Model file for the job. Use its own axes, mm. A direction names the side the tool comes from. Coordinates: 2 decimals unless noted, no trailing zeros. Order: outer loops, then holes, each group sorted by start corner. A loop starts at its lowest first (then second) coordinate and runs counter-clockwise, first axis right, second up. Notation, with made-up numbers: (70.25, -7) -> (78.25, -7) arc R21 ccw to (78.25, 28) -> close; hole circle Ø1 at (28.25, 56.25). An arc over 180 degrees is marked (long way). Return JSON: item names as keys, results as strings. Group by question number.
1) Cut at B-B (x = 26). Write the cut outline in (y, z), and give its area (3 significant figures).
2) Which spindle directions (+Z, -Z, +X, -X, +Y, -Y) get a long thin tool onto all of the face, cutting with end or side? Do faces 1 (the cylindrical face through (5.697, 48.008, 2.877)), 2 (the flat face through (1.016, 58, -11)), 3 (the flat face through (10, 11.43, -7)). Say none if no direction does.
3) Pull direction X, two halves, no side cores. Call faces 4 (the cylindrical face through (5.948, 49.785, -11.13)), 5 (the flat face through (-10, 61.976, 0)), 6 (the flat face through (37.846, 24, -2)): +X half, -X half, draft (parallel to the pull), parting line (faces both ways), or undercut.
4) Flat gauge pins, fed straight in: pin 1 (2 mm diameter, centred on x = 33.09, y = 58.03, fed in from -Z); pin 2 (3 mm diameter, centred on y = 7.5, z = -16, fed in from -X); pin 3 (2.5 mm diameter, centred on x = 13, z = 13, fed in from +Y); pin 4 (2.5 mm diameter, centred on x = -1.5, z = -7, fed in from +Y). Where does each tip first touch, or does it go through?
5) Cut at A-A (y = 26). Write the cut outline in (x, z).
6) Probe line 1 (Z direction, x = 24.5, y = 37); line 2 (X direction, y = 57, z = 4.5); line 3 (Y direction, x = -14.5, z = 12). List the from-to ranges inside material, lowest first.
from build123d import *

# Parameters (mm, degrees)
SKETCH1_W                       = 56.896
SKETCH1_H                       = 9.525
BOSS_EXTRUDE1_DEPTH             = 61.976
SKETCH2_R                       = 13.3985
CUT_EXTRUDE1_DEPTH              = 5.8801
CUT_EXTRUDE1_DRAFT              = -50
SKETCH5_W                       = 56.896
SKETCH5_H                       = 11.43
BOSS_EXTRUDE2_DEPTH             = 7.62
TAP_DRILL_FOR_M3X0_5_TAP3_D     = 2.5
TAP_DRILL_FOR_M3X0_5_TAP3_DEPTH = 25.4
TAP_DRILL_FOR_M3X0_5_TAP3_TIP   = 0.751075774
BOSS_EXTRUDE4_DEPTH             = 56.896
M3_CLEARANCE_HOLE3_D            = 3.7
M3_CLEARANCE_HOLE3_DEPTH        = 25.4
M3_CLEARANCE_HOLE3_TIP          = 1.111592145
SKETCH6_W                       = 56.896
SKETCH6_H                       = 2.54
BOSS_EXTRUDE5_DEPTH             = 50.546
SKETCH24_R                      = 4.826
CUT_EXTRUDE2_DEPTH              = 2.54
SKETCH25_R                      = 6.604
CUT_EXTRUDE3_DEPTH              = 7.366
M3_CLEARANCE_HOLE4_D            = 3.7
M3_CLEARANCE_HOLE4_DEPTH        = 17.272
M3_CLEARANCE_HOLE4_TIP          = 1.111592145


with BuildPart() as part:
    # Sketch1 → Boss-Extrude1 (new body)
    with BuildSketch(Plane(origin=(0, 0, 0), x_dir=(1, 0, 0), z_dir=(0, 1, 0))):
        with Locations((9.398, 0)):
            Rectangle(SKETCH1_W, SKETCH1_H)
    extrude(amount=BOSS_EXTRUDE1_DEPTH)


with BuildPart() as cut_extrude1_tool:
    # Sketch2 → Cut-Extrude1 (with draft: the straight prism first)
    with BuildSketch(Plane(origin=(0, 0, -4.7625), x_dir=(-1, 0, 0), z_dir=(0, 0, -1))):
        with Locations((-5.842, 54.552080914)):
            Circle(SKETCH2_R)
    extrude(amount=-CUT_EXTRUDE1_DEPTH)
    # Cut-Extrude1: the draft: its side faces are tilted about the plane it starts from
    cut_extrude1_sides = [cut_extrude1_tool.faces().sort_by_distance(p)[0] for p in [
        (19.2405, 54.552080914, -1.82245),
    ]]
    draft(cut_extrude1_sides, Plane(origin=(0, 0, -4.7625), x_dir=(-1, 0, 0), z_dir=(0, 0, -1)), CUT_EXTRUDE1_DRAFT)


with BuildPart() as part_1:
    add(part.part)

    # Cut-Extrude1: cut by cut_extrude1_tool
    add(cut_extrude1_tool.part, mode=Mode.SUBTRACT)

    # Sketch5 → Boss-Extrude2 (add)
    with BuildSketch(Plane(origin=(0, 0, -4.7625), x_dir=(-1, 0, 0), z_dir=(0, 0, -1))):
        with Locations((-9.398, 5.715)):
            Rectangle(SKETCH5_W, SKETCH5_H)
    extrude(amount=BOSS_EXTRUDE2_DEPTH)

    # Tap Drill for M3x0.5 Tap3
    with Locations(Plane(origin=(0, 11.43, 0), x_dir=(1, 0, 0), z_dir=(0, 1, 0))):
        with Locations((31.496, 7.3025)):
            Hole(TAP_DRILL_FOR_M3X0_5_TAP3_D / 2, depth=TAP_DRILL_FOR_M3X0_5_TAP3_DEPTH)
            with Locations((0, 0, -(TAP_DRILL_FOR_M3X0_5_TAP3_DEPTH + TAP_DRILL_FOR_M3X0_5_TAP3_TIP / 2))):  # 118° drill point
                Cone(0, TAP_DRILL_FOR_M3X0_5_TAP3_D / 2, TAP_DRILL_FOR_M3X0_5_TAP3_TIP, mode=Mode.SUBTRACT)

    # Sketch19 → Boss-Extrude4 (add)
    with BuildSketch(Plane(origin=(37.846, 0, 0), x_dir=(0, 0, -1), z_dir=(1, 0, 0))):
        with BuildLine():
            Line((12.3825, 8.89), (12.3825, 0))
            Line((12.3825, 0), (28.2575, 0))
            Line((28.2575, 0), (28.2575, 6.35))
            Line((28.2575, 6.35), (14.9225, 6.35))
            ThreePointArc((14.9225, 6.35), (13.126448776, 7.093948776), (12.3825, 8.89))
        make_face()
        with BuildLine():
            Line((-14.9225, 0), (-4.7625, 0))
            Line((-4.7625, 0), (-4.7625, 8.2423))
            ThreePointArc((-4.7625, 8.2423), (-5.316741838, 6.904241838), (-6.6548, 6.35))
            Line((-6.6548, 6.35), (-14.9225, 6.35))
            Line((-14.9225, 6.35), (-14.9225, 0))
        make_face()
    extrude(amount=-BOSS_EXTRUDE4_DEPTH)

    # M3 Clearance Hole3
    with Locations(Plane(origin=(0, 0, 0), x_dir=(-1, 0, 0), z_dir=(0, -1, 0))):
        with Locations((-31.496, -11.1125), (-31.496, 19.3675)):
            Hole(M3_CLEARANCE_HOLE3_D / 2, depth=M3_CLEARANCE_HOLE3_DEPTH)
            with Locations((0, 0, -(M3_CLEARANCE_HOLE3_DEPTH + M3_CLEARANCE_HOLE3_TIP / 2))):  # 118° drill point
                Cone(0, M3_CLEARANCE_HOLE3_D / 2, M3_CLEARANCE_HOLE3_TIP, mode=Mode.SUBTRACT)

    # Sketch6 → Boss-Extrude5 (add)
    with BuildSketch(Plane(origin=(0, 11.43, 0), x_dir=(1, 0, 0), z_dir=(0, 1, 0))):
        with Locations((9.398, 11.1125)):
            Rectangle(SKETCH6_W, SKETCH6_H)
    extrude(amount=BOSS_EXTRUDE5_DEPTH)

    # Sketch24 → Cut-Extrude2 (cut)
    with BuildSketch(Plane(origin=(0, 0, -12.3825), x_dir=(-1, 0, 0), z_dir=(0, 0, -1))):
        with BuildLine():
            ThreePointArc((-10.668, 54.61), (-5.842, 59.436), (-1.016, 54.61))
            Line((-1.016, 54.61), (-1.016, 61.976))
            Line((-1.016, 61.976), (-10.668, 61.976))
            Line((-10.668, 61.976), (-10.668, 54.61))
        make_face()
        with Locations((-5.842, 54.61)):
            Circle(SKETCH24_R)
    extrude(amount=-CUT_EXTRUDE2_DEPTH, mode=Mode.SUBTRACT)

    # Sketch25 → Cut-Extrude3 (cut)
    with BuildSketch(Plane.XY.offset(4.7625)):
        with BuildLine():
            ThreePointArc((-0.762, 54.61), (5.842, 61.214), (12.446, 54.61))
            Line((12.446, 54.61), (12.446, 61.976))
            Line((12.446, 61.976), (-0.762, 61.976))
            Line((-0.762, 61.976), (-0.762, 54.61))
        make_face()
        with Locations((5.842, 54.61)):
            Circle(SKETCH25_R)
    extrude(amount=-CUT_EXTRUDE3_DEPTH, mode=Mode.SUBTRACT)

    # M3 Clearance Hole4
    with Locations(Plane(origin=(0, 0, -12.3825), x_dir=(-1, 0, 0), z_dir=(0, 0, -1))):
        with Locations((-33.09066659, 58.02989171), (12.806122092, 58.02989171)):
            Hole(M3_CLEARANCE_HOLE4_D / 2, depth=M3_CLEARANCE_HOLE4_DEPTH)
            with Locations((0, 0, -(M3_CLEARANCE_HOLE4_DEPTH + M3_CLEARANCE_HOLE4_TIP / 2))):  # 118° drill point
                Cone(0, M3_CLEARANCE_HOLE4_D / 2, M3_CLEARANCE_HOLE4_TIP, mode=Mode.SUBTRACT)


solid = part_1.part
Answers below:
{
 "1": {"outline": "(0, -28.26) -> (6.35, -28.26) -> (6.35, -14.92) arc R2.54 cw to (8.89, -12.38) -> (61.98, -12.38) -> (61.98, -9.84) -> (11.43, -9.84) -> (11.43, -4.76) -> (61.98, -4.76) -> (61.98, 4.76) -> (8.24, 4.76) arc R1.89 cw to (6.35, 6.65) -> (6.35, 14.92) -> (0, 14.92) -> close", "area": "973 mm^2"},
 "2": {"face 1": "+Z, +Y", "face 2": "+Z, -Z, +Y", "face 3": "+X, -X, +Y"},
 "3": {"face 4": "undercut", "face 5": "draft", "face 6": "+X half"},
 "4": {"pin 1": "passes through", "pin 2": "stops at x = -19.05", "pin 3": "stops at y = 6.35", "pin 4": "stops at y = 11.43"},
 "5": {"outline": "(-19.05, -12.38) -> (37.85, -12.38) -> (37.85, -9.84) -> (-19.05, -9.84) -> close; (-19.05, -4.76) -> (37.85, -4.76) -> (37.85, 4.76) -> (-19.05, 4.76) -> close"},
 "6": {"line 1": "z = -12.38 to -9.84, -4.76 to 4.76", "line 2": "x = -19.05 to -14.34, -11.27 to -0.76, 12.45 to 31.55, 34.63 to 37.85", "line 3": "y = 0 to 6.35"}
}
